from build123d import *


with BuildPart() as part:
    # Sketch1 → Revolve1 (revolve)
    with BuildSketch(Plane(origin=(0, 0, 0), x_dir=(1, 0, 0), z_dir=(0, 1, 0))):
        Polygon((0, 0), (88.9, 0), (88.9, -6.35), (77.6478, -6.35), (77.6478, -3.7084), (73.025, -3.7084), (73.025, -6.35), (69.723, -6.35), (69.723, -11.176), (66.6242, -11.176), (66.6242, -15.113), (69.723, -15.113), (69.723, -18.288), (66.6242, -18.288), (66.6242, -22.225), (69.723, -22.225), (69.723, -25.4), (63.4492, -25.4), (63.4492, -3.81), (0, -3.81), align=None)
    revolve(axis=Axis((0, 0, 0), (0, 0, 1)))


solid = part.part
Build history of the part. All positions in model axes, mm. A direction names the side the tool comes from. Round coordinates to 2 decimals unless told otherwise and drop trailing zeros. Write item = value, one per line.
(1) Probe L1, parallel to Y at x = 0, z = 5.25 (3 decimals); L2, parallel to Z at x = 49, y = 46.5 (3 decimals); L3, parallel to Y at x = 0, z = 9. List the from-to ranges inside material, lowest first.
Answer:
L1 = -88.9 to -77.648, -73.025 to -63.449, 63.449 to 73.025, 77.648 to 88.9
L2 = 0 to 11.176, 15.113 to 18.288, 22.225 to 25.4
L3 = -69.72 to -63.45, 63.45 to 69.72
(2) Tool access for faces 5 (the face through (0, -79, 6.35)), 6 (the face through (1, 1, 0)), 7 (the face through (56.5, -35.8, 18.288)): list every direction of +Z, -Z, +X, -X, +Y, -Y with a clear straight run to the whole face (end or side of a thin tool).
Answer:
face_5 = +Z
face_6 = -Z, +X, -X, +Y, -Y
face_7 = none
(3) Two-plate mould, pull along Z, no slides. Class faces 1 (the face through (15, -62, 25.4)), 2 (the face through (-56.5, -35.8, 15.113)), 3 (the face through (-52.9, -40.5, 20.3)), 4 (the face through (-50.35, -38.61, 14.45)): pulls with the +Z half, pulls with the -Z half, needs draft (parallel to the pull), parting line crosses it, or undercut.
Answer:
face_1 = pulls with the +Z half
face_2 = undercut
face_3 = undercut
face_4 = needs draft
(4) Flat gauge pins, fed straight in: pin 1 (5 mm diameter, centred on y = 64.5, z = 15, fed in from +X); pin 2 (2 mm diameter, centred on y = 23, z = 17, fed in from -X); pin 3 (8 mm diameter, centred on x = -59.5, z = 5, fed in from -Y). Where does each tip first touch, or does it go through?
Answer:
pin_1 = 31.89
pin_2 = -66.16
pin_3 = -69.45
